from build123d import *

# Parameters (mm, degrees)
SKETCH3_W              = 16.6
SKETCH3_H              = 25
F_25_0MM_DOWEL_HOLE2_D = 33.2


with BuildPart() as part:
    # Sketch1 → Revolve1 (revolve)
    with BuildSketch(Plane.XY, mode=Mode.PRIVATE) as revolve1_sk:
        Polygon((20, -30), (20, -40), (0, -40), (0, 40), (20, 40), (20, 30), (25, 30), (25, -30), align=None)
    revolve(revolve1_sk.sketch.rotate(Axis((0, 40, 0), (0, -1, 0)), 90), axis=Axis((0, 40, 0), (0, -1, 0)))

    # Sketch3 → Ø1.0mm Dowel Hole1 (revolve, cut)
    with BuildSketch(Plane.ZX):
        with Locations((8.3, 12.5)):
            Rectangle(SKETCH3_W, SKETCH3_H)
    revolve(axis=Axis((-6.35, 0, 0), (1, 0, 0)), mode=Mode.SUBTRACT)

    # Ø25.0mm Dowel Hole2 (through all)
    with Locations(Plane(origin=(0, 0, 0), x_dir=(0, 0, -1), z_dir=(1, 0, 0))):
        with Locations((0, 0)):
            Hole(F_25_0MM_DOWEL_HOLE2_D / 2)


solid = part.part
Build history of the part. All positions in model axes, mm. A direction names the side the tool comes from. Give positions to 0.01 mm unless a question says otherwise; leave off trailing zeros. Order: outer loops, then holes, each group sorted by start corner. A loop starts at its lowest first (then second) coordinate and runs counter-clockwise, first axis right, second up. Notation, with made-up numbers: M -11,-33 L 32,-33 A24 ccw 32,-8 Z; hole C 6.5,22 d5. An arc over 180 degrees is marked long. Use one line per item in the form item = value.
1) Two-plate mould, pull along Z, no slides. Class faces 1 (the face through (0, 40, 0)), 2 (the face through (-0.88, -35.07, -19.98)), 3 (the face through (-0.35, 4.986, 15.833)): released by +Z, released by -Z, zero draft, split by the parting line, or undercut.
Calculated:
face_1 = zero draft
face_2 = split by the parting line
face_3 = undercut
2) Drop flat-ended pins along their axis: pin 1 (1 mm diameter, centred on x = -18, z = -13, fed in from -Y); pin 2 (1 mm diameter, centred on x = 19.5, y = -28.5, fed in from +Z); pin 3 (6 mm diameter, centred on y = -29.5, z = 2, fed in from -X). Give the stop position or say it passes through.
Calculated:
pin_1 = -30
pin_2 = 16.25
pin_3 = -25
3) Saw through at C-C (x = -15). Give the cut face in (y, z), plus the area to 3 significant figures.
Calculated:
outline = M -40,-13.23 L -30,-13.23 L -30,-20 L 30,-20 L 30,-13.23 L 40,-13.23 L 40,13.23 L 30,13.23 L 30,20 L -30,20 L -30,13.23 L -40,13.23 Z; hole C 0,0 d33.2
area = 2,060 mm2
4) Saw through at D-D (y = 1.5). Give the cut face in (x, z), plus the area to 3 significant figures.
Calculated:
outline = M -18.75,-16.53 A25 ccw 18.75,-16.53 Z; M -18.75,16.53 L 18.75,16.53 A25 ccw Z
area = 440 mm2
5) Saw through at A-A (z = 0). Give the cut face in (x, y).
Calculated:
outline = M -25,-30 L -20,-30 L -20,-40 L 20,-40 L 20,-30 L 25,-30 L 25,-16.6 L -25,-16.6 Z; M -25,16.6 L 25,16.6 L 25,30 L 20,30 L 20,40 L -20,40 L -20,30 L -25,30 Z
6) Probe probe 1 along Y at (x, z) = (6, 0); probe 2 along Z at (x, y) = (6, 0); probe 3 along Z at (x, y) = (-5, 0). List the from-to ranges inside material, lowest first.
Calculated:
probe_1 = -40 to -16.6, 16.6 to 40
probe_2 = -24.27 to -16.6, 16.6 to 24.27
probe_3 = -24.49 to -16.6, 16.6 to 24.49
7) Tool access for faces 4 (the face through (-0.88, 34.93, -19.98)), 5 (the face through (-17, -30, -11)), 6 (the face through (-1.099, -0.42, -24.976)): list every direction of +Z, -Z, +X, -X, +Y, -Y with a clear straight run to the whole face (end or side of a thin tool).
Calculated:
face_4 = +Y
face_5 = -Y
face_6 = +Y, -Y
8) Saw through at B-B (x = -21). Give the cut face in (y, z).
Calculated:
outline = M -30,-13.56 L -9.57,-13.56 A16.6 cw -9.57,13.56 L -30,13.56 Z; M 9.57,-13.56 L 30,-13.56 L 30,13.56 L 9.57,13.56 A16.6 cw Z
